Geometry: final body of the model. Coordinates: model frame, mm. A direction names the side the tool comes from. Coordinates: 2 decimals unless noted, no trailing zeros. Loops run counter-clockwise (first coordinate to the right, second up) from the corner with the lowest first, then second, coordinate; pieces in that order, holes last. Notation, with made-up numbers: (-14, 88) -> (-7, 88) arc R16 cw to (-7, 103) -> close; hole circle Ø5 at (22, -30.75). An arc over 180 degrees is marked (long way). One line per item, written item: value. Start each with the question number.
Item 1: Contact query for a flat-ended pin moving along its axis: pin 1 Ø1.6 at (x, z) = (-48.63, 14.2) entering from +Y. Output: stop coordinate, or through.
Item 2: Section query B-B on z = -13. Return loops of the section in (x, y).
Item 3: Section query A-A on y = 0.45. Give the number of separate pieces and of enclosed holes in the cut face, then the cut area to 3 significant figures.
Item 4: Ray query, probe 1 along X at (y, z) = (1.65, 21.5); probe 2 along Z at (x, y) = (8, 1.2); probe 3 along Z at (x, y) = (50.5, 1.8). Return the intervals inside material, ascending. Write a range as from..to.
Item 5: Mould query, pull axis Z, two halves, no side actions, for faces 3 (the flat face through (-23.147, 1.479, 46.296)), 4 (the flat face through (0, 0, -1)). Classes: +Z half, -Z half, draft (parallel to the pull), parting line (faces both ways), or undercut.
Item 6: Set-up query: faces 1 (the flat face through (-49.632, 1.479, -24.138)), 2 (the flat face through (2.966, 1.479, 31.375)). Return all of +Z, -Z, +X, -X, +Y, -Y with unobstructed straight access to the full face (end or side cutting, diameter ignored); none if empty.
from build123d import *

# Parameters (mm, degrees)
CROQUIS1_R              = 1
CROQUIS1_R_2            = 1.5
CROQUIS1_R_3            = 3
SALIENTE_EXTRUIR1_DEPTH = 3


with BuildPart() as part:
    # Croquis1 → Saliente-Extruir1 (new body)
    with BuildSketch(Plane(origin=(0, 0, 0), x_dir=(1, 0, 0), z_dir=(0, 1, 0))):
        with BuildLine():
            Line((-54.220965168, 25.692157096), (-44.912977861, 22.539152286))
            Line((-44.912977861, 22.539152286), (-57.890214642, -15.770955858))
            ThreePointArc((-57.890214642, -15.770955858), (-19.250061989, -56.828119038), (36.387638976, -47.706810098))
            Line((36.387638976, -47.706810098), (49.364875757, -9.396701954))
            Line((49.364875757, -9.396701954), (58.672863064, -12.549706764))
            ThreePointArc((58.672863064, -12.549706764), (19.250061989, 56.828119038), (-54.220965168, 25.692157096))
        make_face()
        with Locations(Location((-48.627206238, -14.202170607, 0), (0, 0, 270))):
            Circle(CROQUIS1_R, mode=Mode.SUBTRACT)
        with Locations(Location((-43.012604824, 2.372697446, 0), (0, 0, 270))):
            Circle(CROQUIS1_R, mode=Mode.SUBTRACT)
        with Locations(Location((35.599626512, -24.256554973, 0), (0, 0, 90))):
            Circle(CROQUIS1_R, mode=Mode.SUBTRACT)
        with Locations(Location((29.985025098, -40.831423025, 0), (0, 0, 90))):
            Circle(CROQUIS1_R, mode=Mode.SUBTRACT)
        with Locations(Location((-24.357390716, 49.312447896, 0), (0, 0, 270))):
            Circle(CROQUIS1_R_2, mode=Mode.SUBTRACT)
        with Locations(Location((49.312447896, 24.357390716, 0), (0, 0, 270))):
            Circle(CROQUIS1_R_2, mode=Mode.SUBTRACT)
        with Locations(Location((24.357390716, -49.312447896, 0), (0, 0, 270))):
            Circle(CROQUIS1_R_2, mode=Mode.SUBTRACT)
        with Locations(Location((-49.312447896, -24.357390716, 0), (0, 0, 270))):
            Circle(CROQUIS1_R_2, mode=Mode.SUBTRACT)
        with Locations(Location((-32.085428511, 7.800903466, 0), (0, 0, 270))):
            Circle(CROQUIS1_R_2, mode=Mode.SUBTRACT)
        with Locations(Location((30.220997798, -13.304890445, 0), (0, 0, 90))):
            Circle(CROQUIS1_R_2, mode=Mode.SUBTRACT)
        with Locations(Location((45.752512271, 32.552062119, 0), (0, 0, 270))):
            Circle(CROQUIS1_R_2, mode=Mode.SUBTRACT)
        with Locations(Location((-16.551981469, 53.657201388, 0), (0, 0, 270))):
            Circle(CROQUIS1_R_2, mode=Mode.SUBTRACT)
        with Locations(Location((35.282961094, 1.644894083, 0), (0, 0, 270))):
            Circle(CROQUIS1_R_2, mode=Mode.SUBTRACT)
        with Locations(Location((-27.019600078, 22.74937871, 0), (0, 0, 270))):
            Circle(CROQUIS1_R_2, mode=Mode.SUBTRACT)
        with Locations(Location((8.315068564, 55.715649476, 0), (0, 0, 270))):
            Circle(CROQUIS1_R_2, mode=Mode.SUBTRACT)
        with Locations(Location((27.25777491, 49.298962147, 0), (0, 0, 270))):
            Circle(CROQUIS1_R_2, mode=Mode.SUBTRACT)
        with Locations(Location((20.841087581, 30.356255801, 0), (0, 0, 270))):
            Circle(CROQUIS1_R_2, mode=Mode.SUBTRACT)
        with Locations(Location((1.898381235, 36.77294313, 0), (0, 0, 270))):
            Circle(CROQUIS1_R_2, mode=Mode.SUBTRACT)
        with Locations(Location((-37.36617256, 33.867636702, 0), (0, 0, 270))):
            Circle(CROQUIS1_R_3, mode=Mode.SUBTRACT)
        Polygon((31.329833693, -24.393920483), (26.838152562, -37.653814925), (19.261070024, -35.087139993), (23.752751155, -21.827245551), align=None, mode=Mode.SUBTRACT)
        with BuildLine():
            Line((-2.242259213, -26.971782408), (9.596932254, -30.982211989))
            ThreePointArc((9.596932254, -30.982211989), (10.379806837, -32.567178833), (8.79483686, -33.350047072))
            Line((8.79483686, -33.350047072), (-3.029342655, -29.344597153))
            ThreePointArc((-3.029342655, -29.344597153), (-3.829733257, -27.762151967), (-2.242259213, -26.971782408))
        make_face(mode=Mode.SUBTRACT)
        with BuildLine():
            Line((4.686376156, -0.283162711), (20.314364649, -5.577019828))
            ThreePointArc((20.314364649, -5.577019828), (22.050140606, -4.71913044), (21.192235329, -2.983362336))
            Line((21.192235329, -2.983362336), (5.531032931, 2.233688827))
            ThreePointArc((5.531032931, 2.233688827), (3.853823576, 1.396401808), (4.686376156, -0.283162711))
        make_face(mode=Mode.SUBTRACT)
        Polygon((12.827287772, -26.900405501), (14.721558407, -27.542074234), (20.481483355, -10.538196491), (18.58721272, -9.896527758), align=None, mode=Mode.SUBTRACT)
        Polygon((-44.196996235, -13.591237439), (-36.619913697, -16.15791237), (-32.128232566, -2.898017928), (-39.705315105, -0.331342996), align=None, mode=Mode.SUBTRACT)
        with BuildLine():
            Line((-27.816509098, -44.714655504), (-18.345155925, -47.922999169))
            ThreePointArc((-18.345155925, -47.922999169), (-16.760193821, -47.14012298), (-17.543070009, -45.555160876))
            Line((-17.543070009, -45.555160876), (-27.014423182, -42.346817211))
            ThreePointArc((-27.014423182, -42.346817211), (-28.599385287, -43.129693399), (-27.816509098, -44.714655504))
        make_face(mode=Mode.SUBTRACT)
        Polygon((-20.550996192, 4.141245501), (-22.445266826, 4.782914234), (-33.101695464, -26.675934859), (-31.207424829, -27.317603592), align=None, mode=Mode.SUBTRACT)
        with BuildLine():
            Line((-35.583265447, -38.380985707), (-32.483875307, -39.430878847))
            ThreePointArc((-32.483875307, -39.430878847), (-31.034585959, -38.71501686), (-31.750447946, -37.265727512))
            Line((-31.750447946, -37.265727512), (-34.849838086, -36.215834372))
            ThreePointArc((-34.849838086, -36.215834372), (-36.299127434, -36.931696359), (-35.583265447, -38.380985707))
        make_face(mode=Mode.SUBTRACT)
        Polygon((-1.74088879, -2.230525018), (-12.397317428, -33.68937411), (-15.282344998, -42.206265656), (-17.176615633, -41.564596923), (-14.291588062, -33.047705377), (-3.635159425, -1.588856285), align=None, mode=Mode.SUBTRACT)
        Polygon((-35.216834792, 17.75393043), (-32.65015986, 25.331012969), (-36.438701129, 26.614350435), (-39.005376061, 19.037267896), align=None, mode=Mode.SUBTRACT)
        with BuildLine():
            Line((-7.485817773, -50.925076541), (-3.314971008, -38.612317416))
            ThreePointArc((-3.314971008, -38.612317416), (-2.810697341, -38.036561821), (-2.047001325, -37.986016465))
            Line((-2.047001325, -37.986016465), (5.530081214, -40.552691397))
            ThreePointArc((5.530081214, -40.552691397), (6.105836809, -41.056965065), (6.156382165, -41.820661081))
            Line((6.156382165, -41.820661081), (1.9855354, -54.133420206))
            ThreePointArc((1.9855354, -54.133420206), (1.481261732, -54.709175801), (0.717565717, -54.759721157))
            Line((0.717565717, -54.759721157), (-6.859516822, -52.193046225))
            ThreePointArc((-6.859516822, -52.193046225), (-7.435272417, -51.688772557), (-7.485817773, -50.925076541))
        make_face(mode=Mode.SUBTRACT)
        with BuildLine():
            Line((-1.151422367, -23.751522329), (10.6877691, -27.76195191))
            ThreePointArc((10.6877691, -27.76195191), (11.470645288, -29.346914015), (9.885683184, -30.129790204))
            Line((9.885683184, -30.129790204), (-1.953508283, -26.119360623))
            ThreePointArc((-1.953508283, -26.119360623), (-2.736384471, -24.534398518), (-1.151422367, -23.751522329))
        make_face(mode=Mode.SUBTRACT)
        with BuildLine():
            Line((3.691828695, -3.220011933), (19.319561431, -8.51377898))
            ThreePointArc((19.319561431, -8.51377898), (20.904523535, -7.730902791), (20.121647347, -6.145940687))
            Line((20.121647347, -6.145940687), (4.493914611, -0.85217364))
            ThreePointArc((4.493914611, -0.85217364), (2.908952507, -1.635049828), (3.691828695, -3.220011933))
        make_face(mode=Mode.SUBTRACT)
        with BuildLine():
            Line((-20.18129085, 7.087192335), (-18.287020215, 6.445523602))
            ThreePointArc((-18.287020215, 6.445523602), (-17.571158228, 4.996234254), (-19.020447577, 4.280372267))
            Line((-19.020447577, 4.280372267), (-20.914718212, 4.922041))
            ThreePointArc((-20.914718212, 4.922041), (-21.630580198, 6.371330349), (-20.18129085, 7.087192335))
        make_face(mode=Mode.SUBTRACT)
        with BuildLine():
            Line((-4.03263369, 1.616966387), (-2.138363055, 0.975297654))
            ThreePointArc((-2.138363055, 0.975297654), (-1.422501068, -0.473991695), (-2.871790417, -1.189853682))
            Line((-2.871790417, -1.189853682), (-4.766061052, -0.548184949))
            ThreePointArc((-4.766061052, -0.548184949), (-5.481923038, 0.9011044), (-4.03263369, 1.616966387))
        make_face(mode=Mode.SUBTRACT)
        with BuildLine():
            Line((-19.544125985, -41.400519554), (-16.806910291, -42.327729053))
            ThreePointArc((-16.806910291, -42.327729053), (-16.091048304, -43.777018402), (-17.540337653, -44.492880389))
            Line((-17.540337653, -44.492880389), (-20.277553347, -43.56567089))
            ThreePointArc((-20.277553347, -43.56567089), (-20.993415333, -42.116381541), (-19.544125985, -41.400519554))
        make_face(mode=Mode.SUBTRACT)
        with BuildLine():
            Line((-12.233875617, 5.870044257), (-4.656823255, 3.303379547))
            ThreePointArc((-4.656823255, 3.303379547), (-3.514904412, 3.869424877), (-4.084170263, 5.009741653))
            Line((-4.084170263, 5.009741653), (-11.675589384, 7.533597029))
            ThreePointArc((-11.675589384, 7.533597029), (-12.784164712, 6.980177058), (-12.233875617, 5.870044257))
        make_face(mode=Mode.SUBTRACT)
        with BuildLine():
            Line((-16.734038691, 7.116277585), (-4.860468149, 3.108408302))
            ThreePointArc((-4.860468149, 3.108408302), (-4.389721673, 2.157935917), (-5.340194058, 1.687189441))
            Line((-5.340194058, 1.687189441), (-17.213764599, 5.695058723))
            ThreePointArc((-17.213764599, 5.695058723), (-17.684511076, 6.645531108), (-16.734038691, 7.116277585))
        make_face(mode=Mode.SUBTRACT)
    extrude(amount=SALIENTE_EXTRUIR1_DEPTH)


solid = part.part
Reply:
1. pin 1: passes through
2. outline: (-48.14, 0) -> (58.57, 0) -> (58.57, 3) -> (-48.14, 3) -> close
3. separate pieces: 1
3. enclosed holes: 37
3. area: 9,700 mm²
4. probe 1: x = -56.02..-31.35, -29.24..-10.38, -8.27..14.66, 16.77..45.26
4. probe 2: z = -59.46..-57.18, -54.25..-1.41, 1.41..2.04, 4.68..26.85, 29.49..30.44, 33.08..59.46
4. probe 3: z = -32.4..-25.27, -23.44..9.78
5. face 3: undercut
5. face 4: draft
6. face 1: -X, +Y, -Y
6. face 2: +Y, -Y
